The listing builds one solid part. Answer for the finished solid, in the listing's coordinates (mm). A direction names the side the tool comes from. Coordinates: 2 decimals unless noted, no trailing zeros. Order: outer loops, then holes, each group sorted by start corner. A loop starts at its lowest first (then second) coordinate and runs counter-clockwise, first axis right, second up. Notation, with made-up numbers: M 42,23.5 L 88,23.5 A14 cw 88,50.5 Z; hole C -24.5,12 d2. An arc over 180 degrees is marked long. One line per item, written item: value. Start each with the question number.
Q1. For faces 1 (the flat face through (1157, -31.75, 25)), 2 (the flat face through (1157, -488.95, 25)), determine the directions among +Z, -Z, +X, -X, +Y, -Y from which every point of the face is accessible in a straight line to the end or side of a thin tool.
Q2. The part is cut by section B-B on x = 333.5. Give the vertices of the cut face in (y, z) (3 decimals).
Q3. Straight lines are drawn through the part: line 1 along Y through (x, z) = (190.5, 42.5) (3 decimals); line 2 along Y through (x, z) = (691, 19.5) (3 decimals); line 3 along Z through (x, y) = (933, -579). For each, find the intervals that lie inside material, in ascending order. Write a range as [from, to].
Q4. The part is cut by section C-C on x = 596.5. Give the vertices of the cut face in (y, z) (3 decimals), then the cut area to 3 significant figures.
Q5. The part is cut by section A-A on y = -322. Give the number of separate pieces and of enclosed holes in the cut face, then the cut area to 3 significant figures.
```python
from build123d import *

# Parameters (mm, degrees)
F0_W     = 1524
F0_H     = 1066.8
F0_W_2   = 304.8
F0_H_2   = 1003.3
F0_W_3   = 660.4
F0_H_3   = 31.75
F0_H_4   = 454.025
F0_W_4   = 431.8
F0_H_5   = 44.45
F1_DEPTH = 50.8
F2_R     = 12.7
F3_DEPTH = 406.4
F4_R     = 6.35
F5_DEPTH = 127
F6_T     = -3.175


# Not quite as in the source:
# - a feature names something its author has since deleted; it is built from what else it names


with BuildPart() as f1:
    # F0 (on Top) → F1 (new body)
    with BuildSketch(Plane.XY):
        with Locations((762, -533.4)):
            Rectangle(F0_W, F0_H)
        Polygon((1492.25, -1035.05), (831.85, -1035.05), (831.85, -832.48246), (831.85, -788.03246), (831.85, -581.025), (1492.25, -581.025), (1492.25, -788.03246), (1492.25, -832.48246), align=None, mode=Mode.SUBTRACT)
        Polygon((31.75, -788.03246), (31.75, -31.75), (463.55, -31.75), (463.55, -788.03246), (463.55, -832.48246), (463.55, -1035.05), (31.75, -1035.05), (31.75, -832.48246), align=None, mode=Mode.SUBTRACT)
        with Locations((647.7, -533.4)):
            Rectangle(F0_W_2, F0_H_2, mode=Mode.SUBTRACT)
        with Locations((1162.05, -533.4)):
            Rectangle(F0_W_3, F0_H_3, mode=Mode.SUBTRACT)
        with Locations((1162.05, -258.7625)):
            Rectangle(F0_W_3, F0_H_4, mode=Mode.SUBTRACT)
        with Locations((247.65, -810.25746)):
            Rectangle(F0_W_4, F0_H_5)
        with Locations((1162.05, -810.25746)):
            Rectangle(F0_W_3, F0_H_5)
    extrude(amount=F1_DEPTH)

    # F2 (on face) → F3 (cut)
    with BuildSketch(Plane(origin=(463.55, 0, 0), x_dir=(0, -1, 0), z_dir=(-1, 0, 0))):
        with Locations((381, 25.4)):
            Circle(F2_R)
        with Locations((685.8, 25.4)):
            Circle(F2_R)
    extrude(amount=-F3_DEPTH, mode=Mode.SUBTRACT)

    # F4 (on face) → F5 (cut)
    with BuildSketch(Plane(origin=(0, -485.775, 0), x_dir=(-1, 0, 0), z_dir=(0, 1, 0))):
        with Locations((-933.45, 25.4)):
            Circle(F4_R)
    extrude(amount=-F5_DEPTH, mode=Mode.SUBTRACT)

    # F6
    f6_openings = [f1.faces().sort_by_distance(p)[0] for p in [
        (815.975, -368.3, 25.4),
        (479.425, -368.3, 25.4),
        (939.8, -565.15, 25.4),
        (939.8, -501.65, 25.4),
    ]]
    offset(amount=F6_T, openings=f6_openings, kind=Kind.INTERSECTION)


solid = f1.part
```
Output:
1. face 1: +Z, -Z
1. face 2: none
2. outline: M -1066.8,0 L -1035.05,0 L -1035.05,50.8 L -1066.8,50.8 Z; M -832.482,0 L -788.032,0 L -788.032,50.8 L -832.482,50.8 Z; M -31.75,0 L 0,0 L 0,50.8 L -31.75,50.8 Z; hole M -1063.625,3.175 L -1038.225,3.175 L -1038.225,47.625 L -1063.625,47.625 Z; hole M -829.307,3.175 L -791.207,3.175 L -791.207,47.625 L -829.307,47.625 Z; hole M -28.575,3.175 L -3.175,3.175 L -3.175,47.625 L -28.575,47.625 Z
3. line 1: y = [-1066.8, -1063.625], [-1038.225, -1035.05], [-832.482, -829.307], [-791.207, -788.032], [-31.75, -28.575], [-3.175, 0]
3. line 2: y = [-1066.8, -1063.625], [-1038.225, -1035.05], [-31.75, -28.575], [-3.175, 0]
3. line 3: z = [0, 19.07], [31.73, 50.8]
4. outline: M -1066.8,0 L -1035.05,0 L -1035.05,50.8 L -1066.8,50.8 Z; M -31.75,0 L 0,0 L 0,50.8 L -31.75,50.8 Z; hole M -1063.625,3.175 L -1038.225,3.175 L -1038.225,47.625 L -1063.625,47.625 Z; hole M -28.575,3.175 L -3.175,3.175 L -3.175,47.625 L -28.575,47.625 Z
4. area: 968 mm^2
5. separate pieces: 4
5. enclosed holes: 4
5. area: 1,940 mm^2
